from build123d import *

# Parameters (mm, degrees)
F0_W       = 59.5488740506
F0_H       = 60
F0_R       = 15
F1_DEPTH   = 125
F2_R       = 15
F1_FACE1_W = 59.5488740506
F1_FACE1_H = 60
F3_DEPTH   = 125.001


with BuildPart() as f1:
    # F0 (on Front) → F1 (new body)
    with BuildSketch(Plane.XZ):
        with Locations((-30.2255629747, 16.9652015452)):
            Rectangle(F0_W, F0_H)
        with Locations((-30.4511259494, 16.9652015452)):
            Circle(F0_R, mode=Mode.SUBTRACT)
        with Locations((-30.4511259494, 16.9652015452)):
            Circle(F0_R)
    extrude(amount=F1_DEPTH)

    # F2 (on face) + F1_face1 (on face) → F3 (cut, through all)
    with BuildSketch(Plane(origin=(0, 0, 0), x_dir=(-1, 0, 0), z_dir=(0, 1, 0))):
        with Locations((30.4511259494, 16.9652015452)):
            Circle(F2_R)
    with BuildSketch(Plane(origin=(-30.2255629747, -125, 16.9652015452), x_dir=(1, 0, 0), z_dir=(0, -1, 0))):
        Rectangle(F1_FACE1_W, F1_FACE1_H)
    extrude(amount=-F3_DEPTH, dir=(0, 1, 0), mode=Mode.SUBTRACT)


solid = f1.part
For this review, take the finished solid that the model builds, in its own axes (mm). Give positions to 0.01 mm unless a question says otherwise; leave off trailing zeros. Loops run counter-clockwise (first coordinate to the right, second up) from the corner with the lowest first, then second, coordinate; pieces in that order, holes last. Notation, with made-up numbers: M -39.5,-5 L -10.5,-5 A23 ccw -10.5,31 Z; hole C 26,75.5 d10. An arc over 180 degrees is marked long. Put each result on its own line as item: value. Start each with the question number.
(1) The part is to be moulded in two halves that separate along X. For faces 1 (the flat face through (-0.451, -62, 17)), 2 (the flat face through (-31, -62, -13.035)), 3 (the cylindrical face through (-37.373, -61.625, 3.658)), 4 (the flat face through (-60, -62, 17)), say which applies: +X half, -X half, draft (parallel to the pull), parting line (faces both ways), or undercut.
(2) Add section C-C, the plane y = -71. Write out the cut boundary in (x, z).
(3) Add section B-B, the plane x = -17. Write out the cut boundary in (y, z).
(4) For pin 1 (5 mm diameter, centred on x = -11, z = 5, fed in from +Y), flat-tipped, find the tip position at first contact; note if it passes through.
(5) Wall thickness on L1, parallel to Z at x = -17, y = -16; L2, parallel to Z at x = -19, y = -69; L3, parallel to X at y = -51.5, z = 16: over which ranges is each line inside the solid? List them lowest first.
(6) Add section A-A, the plane z = 22.5. Write out the cut boundary in (x, y), then the cut area to 3 significant figures.
Result:
1. face 1: +X half
1. face 2: draft
1. face 3: undercut
1. face 4: -X half
2. outline: M -60,-13.03 L -0.45,-13.03 L -0.45,46.97 L -60,46.97 Z; hole C -30.45,16.97 d30
3. outline: M -125,-13.03 L 0,-13.03 L 0,10.33 L -125,10.33 Z; M -125,23.6 L 0,23.6 L 0,46.97 L -125,46.97 Z
4. pin 1: stops at y = 0
5. L1: z = -13.03 to 10.33, 23.6 to 46.97
5. L2: z = -13.03 to 7.28, 26.65 to 46.97
5. L3: x = -60 to -45.42, -15.48 to -0.45
6. outline: M -60,-125 L -44.39,-125 L -44.39,0 L -60,0 Z; M -16.51,-125 L -0.45,-125 L -0.45,0 L -16.51,0 Z
6. area: 3,960 mm^2
